Geometry check sheet. Reference: drawing and pictorial views, mm from the part's lowest x, y, z. Give positions to 0.01 mm unless a question says otherwise; leave off trailing zeros. Loops run counter-clockwise (first coordinate to the right, second up) from the corner with the lowest first, then second, coordinate; pieces in that order, holes last. Notation, with made-up numbers: (55.5, -6.75) -> (108.5, -6.75) arc R25 cw to (108.5, 19.25) -> close; hole circle Ø3 at (-5.5, 12.25). An arc over 180 degrees is marked (long way). Write item = value, one per line. Start each with the question number.
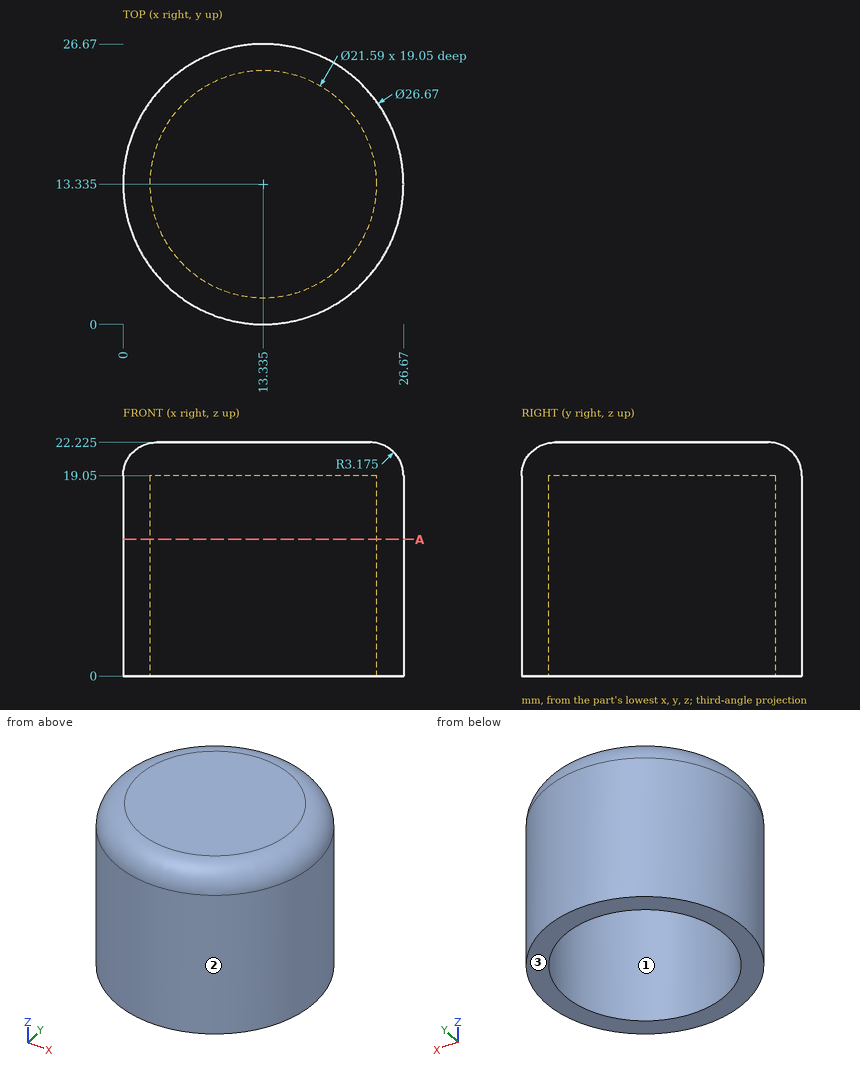
1) Depth check by flat-ended pin: pin 1 Ø4 at (x, y) = (20, 11) entering from -Z; pin 2 Ø4 at (x, z) = (3, 4.5) entering from -Y. Enter the tip coordinate at first touch or a pass-through.
2) Draft check along Y on the marked faces 1, 2 and 3. Enter one of: released by +Y, released by -Y, zero draft, split by the parting line, or undercut.
3) Thickness scan on line 1 (Z direction, x = 11, y = 14.75) (3 decimals); line 2 (Y direction, x = 13, z = 5.75); line 3 (X direction, y = 15.5, z = 2.5). Record the ranges inside material, lowest first.
4) Section check A-A (z = 13). Enter the section's corners in (x, y) (3 decimals).
Check result:
q1.pin_1 = 19.05
q1.pin_2 = 2.93
q2.face_1 = undercut
q2.face_2 = split by the parting line
q2.face_3 = zero draft
q3.line_1 = 19.05 to 22.225
q3.line_2 = 0 to 2.55, 24.12 to 26.67
q3.line_3 = 0.18 to 2.76, 23.91 to 26.49
q4.outline = circle Ø26.67 at (13.335, 13.335); hole circle Ø21.59 at (13.335, 13.335)
